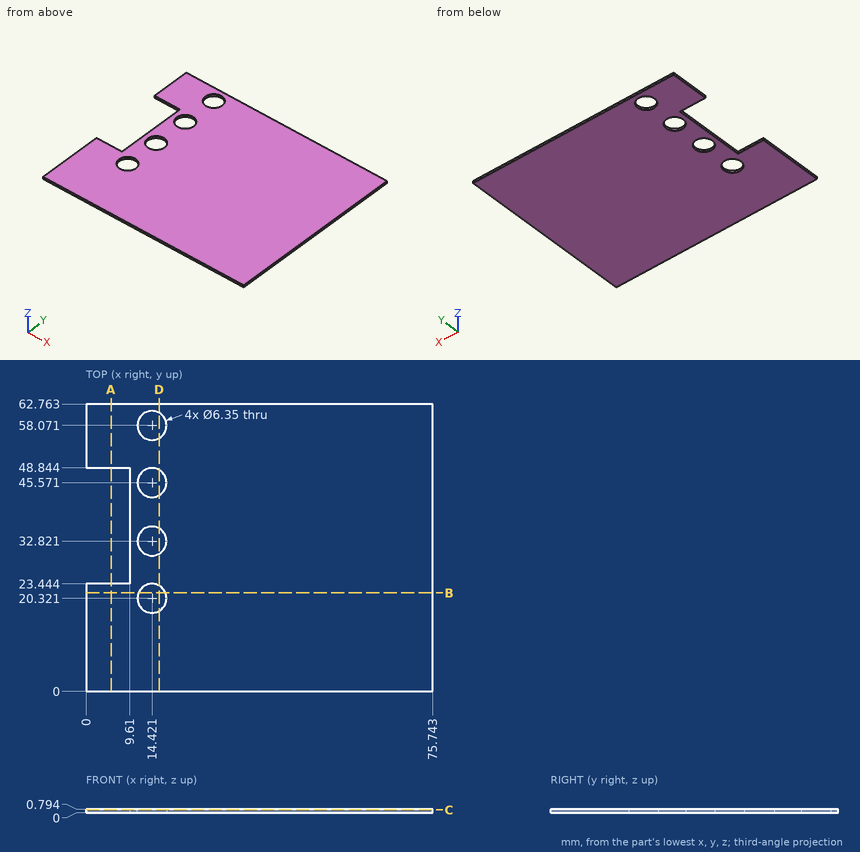
Drawing for the job (mm, zero at the part's lowest x, y, z). Give positions to 0.01 mm unless a question says otherwise; leave off trailing zeros. Loops run counter-clockwise (first coordinate to the right, second up) from the corner with the lowest first, then second, coordinate; pieces in that order, holes last.
1) Band-saw the part on B-B on y = 21.5. List the corners of the cut face in (x, z).
Values follow:
outline: (0, 0) - (11.47, 0) - (11.47, 0.79) - (0, 0.79) - close; (17.37, 0) - (75.74, 0) - (75.74, 0.79) - (17.37, 0.79) - close
2) Drop a flat-ended pin along its axis: P1, Ø5, axis at x = 14.42, y = 20.32, coming from the -Z side. Give the stop position or say it passes through.
Values follow:
P1: passes through
3) Band-saw the part on A-A on x = 5.5. List the corners of the cut face in (y, z) (1 decimal).
Values follow:
outline: (0, 0) - (23.4, 0) - (23.4, 0.8) - (0, 0.8) - close; (48.8, 0) - (62.8, 0) - (62.8, 0.8) - (48.8, 0.8) - close
4) Band-saw the part on C-C on z = 0.65. State how many separate pieces and enclosed holes the cut face has, then the cut area to 3 significant figures.
Values follow:
separate pieces: 1
enclosed holes: 4
area: 4,380 mm2
5) Band-saw the part on D-D on x = 16. List the corners of the cut face in (y, z) (1 decimal).
Values follow:
outline: (0, 0) - (17.6, 0) - (17.6, 0.8) - (0, 0.8) - close; (23.1, 0) - (30.1, 0) - (30.1, 0.8) - (23.1, 0.8) - close; (35.6, 0) - (42.8, 0) - (42.8, 0.8) - (35.6, 0.8) - close; (48.3, 0) - (55.3, 0) - (55.3, 0.8) - (48.3, 0.8) - close; (60.8, 0) - (62.8, 0) - (62.8, 0.8) - (60.8, 0.8) - close
6) Probe line 1 along Y through (x, z) = (11.5, 0.25) (1 decimal); line 2 along Y through (x, z) = (12, 0.2) (1 decimal); line 3 along X through (y, z) = (45.5, 0.35) (1 decimal). List the from-to ranges inside material, lowest first.
Values follow:
line 1: y = 0 to 19.1, 21.6 to 31.6, 34.1 to 44.3, 46.8 to 56.8, 59.3 to 62.8
line 2: y = 0 to 18.3, 22.4 to 30.8, 34.9 to 43.5, 47.6 to 56, 60.1 to 62.8
line 3: x = 9.6 to 11.2, 17.6 to 75.7
